from build123d import *

# Parameters (mm, degrees)
EXTRUDE_1_DEPTH     = 2
SKETCH_2_W          = 46
SKETCH_2_H          = 21
EXTRUDE_2_DEPTH     = 5.5
SKETCH_3_R          = 1.25
CUT_EXTRUDE_1_DEPTH = 8.5
SKETCH_4_R          = 8.5
CUT_EXTRUDE_2_DEPTH = 8.5


with BuildPart() as part:
    # 草图1 → 凸台-拉伸1 (new body)
    with BuildSketch(Plane(origin=(0, 0, 0), x_dir=(1, 0, 0), z_dir=(0, 1, 0))):
        with BuildLine():
            Line((-23, 12.5), (23, 12.5))
            ThreePointArc((23, 12.5), (24.414213562, 11.914213562), (25, 10.5))
            Line((25, 10.5), (25, -10.5))
            ThreePointArc((25, -10.5), (24.414213562, -11.914213562), (23, -12.5))
            Line((23, -12.5), (-23, -12.5))
            ThreePointArc((-23, -12.5), (-24.414213562, -11.914213562), (-25, -10.5))
            Line((-25, -10.5), (-25, 10.5))
            ThreePointArc((-25, 10.5), (-24.414213562, 11.914213562), (-23, 12.5))
        make_face()
    extrude(amount=EXTRUDE_1_DEPTH)

    # 草图2 → 凸台-拉伸2 (add)
    with BuildSketch(Plane(origin=(0, 2, 0), x_dir=(1, 0, 0), z_dir=(0, 1, 0))):
        with BuildLine():
            Line((23, 12.5), (-23, 12.5))
            ThreePointArc((-23, 12.5), (-24.414213562, 11.914213562), (-25, 10.5))
            Line((-25, 10.5), (-25, -10.5))
            ThreePointArc((-25, -10.5), (-24.414213562, -11.914213562), (-23, -12.5))
            Line((-23, -12.5), (23, -12.5))
            ThreePointArc((23, -12.5), (24.414213562, -11.914213562), (25, -10.5))
            Line((25, -10.5), (25, 10.5))
            ThreePointArc((25, 10.5), (24.414213562, 11.914213562), (23, 12.5))
        make_face()
        Rectangle(SKETCH_2_W, SKETCH_2_H, mode=Mode.SUBTRACT)
    extrude(amount=EXTRUDE_2_DEPTH)

    # 草图3 → 切除-拉伸1 (cut, through all)
    with BuildSketch(Plane.XZ):
        with Locations((-21, 8.5)):
            Circle(SKETCH_3_R)
        with Locations((-21, -8.5)):
            Circle(SKETCH_3_R)
        with Locations((21, 8.5)):
            Circle(SKETCH_3_R)
        with Locations((21, -8.5)):
            Circle(SKETCH_3_R)
    extrude(amount=-CUT_EXTRUDE_1_DEPTH, mode=Mode.SUBTRACT)

    # 草图4 → 切除-拉伸2 (cut, through all)
    with BuildSketch(Plane.XZ):
        with Locations((-13.5, 0)):
            Circle(SKETCH_4_R)
        with Locations((13.5, 0)):
            Circle(SKETCH_4_R)
    extrude(amount=-CUT_EXTRUDE_2_DEPTH, mode=Mode.SUBTRACT)


solid = part.part
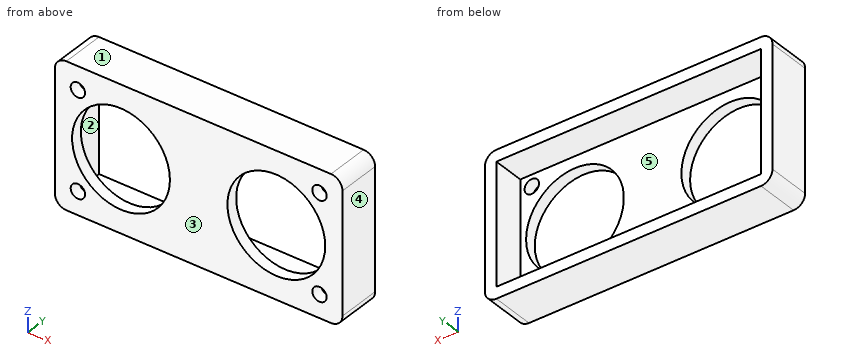
Read the model definition and answer for the solid it produces. Units are mm, in the model's axes. Face numbers are marked on the shaded views. A direction names the side the tool comes from. Round coordinates to 2 decimals unless told otherwise and drop trailing zeros. Order: outer loops, then holes, each group sorted by start corner. A loop starts at its lowest first (then second) coordinate and runs counter-clockwise, first axis right, second up.
1) The part is cut by section A-A on x = 21. Write down the section's boundary in (y, z).
2) Flat-ended cylindrical pins translate along their axes: pin 1 (2 mm diameter, centred on x = -19, z = -5, fed in from -Y); pin 2 (4 mm diameter, centred on x = -4, z = -5, fed in from +Y). Find the tip coordinate at first contact, or state that the pin passes through.
3) Straight lines are drawn through the part: L1, parallel to X at y = 5.75, z = -6; L2, parallel to Z at x = -21, y = 1.55; L3, parallel to Z at x = -13.5, y = 0.9. For each, find the intervals that lie inside material, in ascending order.
4) For the marked faces 4 and 5, determine the directions among +Z, -Z, +X, -X, +Y, -Y from which every point of the face is accessible in a straight line to the end or side of a thin tool.
5) The part is cut by section C-C on x = -13.5. Write down the section's boundary in (y, z), plus the area to 3 significant figures.
6) The part is cut by section D-D on y = 3.5. Write down the section's boundary in (x, z).
7) The part is cut by section B-B on z = 0. Write down the section's boundary in (x, y).
8) The mould has two halves that part along Z. Classify the marked faces 1, 2 and 3: released by +Z, released by -Z, zero draft, split by the parting line, or undercut.
Resolved:
1. outline: (0, -12.5) - (7.5, -12.5) - (7.5, -10.5) - (2, -10.5) - (2, -9.75) - (0, -9.75) - close; (0, -7.25) - (2, -7.25) - (2, -4) - (0, -4) - close; (0, 4) - (2, 4) - (2, 7.25) - (0, 7.25) - close; (0, 9.75) - (2, 9.75) - (2, 10.5) - (7.5, 10.5) - (7.5, 12.5) - (0, 12.5) - close
2. pin 1: passes through
2. pin 2: stops at y = 2
3. L1: x = -25 to -23, 23 to 25
3. L2: z = -12.5 to -9.75, -7.25 to -4, 4 to 7.25, 9.75 to 12.5
3. L3: z = -12.5 to -8.5, 8.5 to 12.5
4. face 4: +Z, -Z, +X, +Y, -Y
4. face 5: +Y
5. outline: (0, -12.5) - (7.5, -12.5) - (7.5, -10.5) - (2, -10.5) - (2, -8.5) - (0, -8.5) - close; (0, 8.5) - (2, 8.5) - (2, 10.5) - (7.5, 10.5) - (7.5, 12.5) - (0, 12.5) - close
5. area: 38.0 mm2
6. outline: (-25, -10.5) arc R2 ccw to (-23, -12.5) - (23, -12.5) arc R2 ccw to (25, -10.5) - (25, 10.5) arc R2 ccw to (23, 12.5) - (-23, 12.5) arc R2 ccw to (-25, 10.5) - close; hole (-23, -10.5) - (23, -10.5) - (23, 10.5) - (-23, 10.5) - close
7. outline: (-25, 0) - (-22, 0) - (-22, 2) - (-23, 2) - (-23, 7.5) - (-25, 7.5) - close; (-5, 0) - (5, 0) - (5, 2) - (-5, 2) - close; (22, 0) - (25, 0) - (25, 7.5) - (23, 7.5) - (23, 2) - (22, 2) - close
8. face 1: released by +Z
8. face 2: undercut
8. face 3: zero draft
